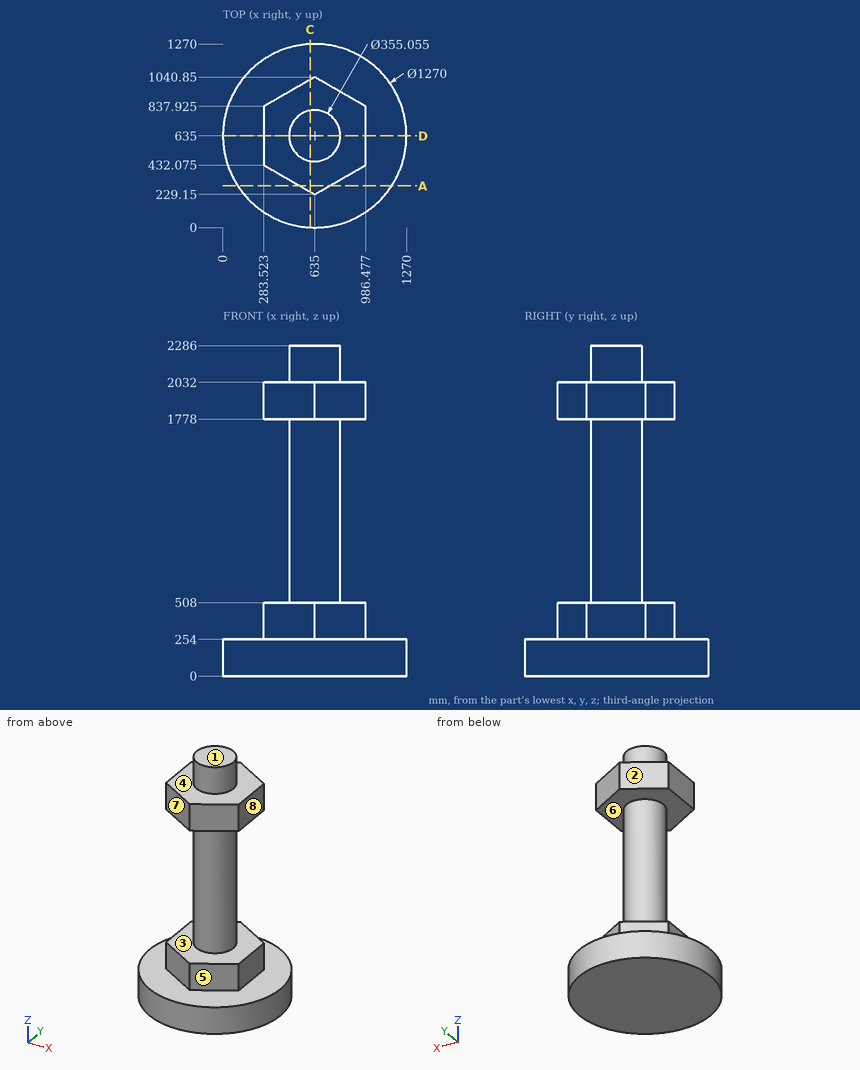
Could you check a few things on this drawing? It's one solid part, dimensions in mm from its lowest x, y, z. A direction names the side the tool comes from. Round coordinates to 2 decimals unless told otherwise and drop trailing zeros. Write each loop counter-clockwise with the first axis right and the second up, starting at its lowest first coordinate (ties: lowest second). Pieces come first, ordered by that corner, then holes. Notation, with made-up numbers: M 18.25,42 L 22.25,42 A11 cw 22.25,50 Z; hole C 41,-11.5 d5. An arc over 180 degrees is marked long. Answer as CSV lines item,"result". Start each with the question number.
1. On a 3-axis mill with a long thin cutter (end or side, diameter ignored), from which of +Z, -Z, +X, -X, +Y, -Y can I reach the whole of each face in a straight line? I mean the marked faces 4, 5, 6, 7 and 8. Say none if no direction works.
2. I need wall thicknesses on probe 1 along Z at (x, y) = (816.5, 820.5); probe 2 along X at (y, z) = (639, 1463.5); probe 3 along X at (y, z) = (620, 1981). Which ranges of each line are inside material? Lowest first, please.
3. I'm going to push a flat-ended pin straight in: pin 1 Ø8 at (x, y) = (299.5, 1017.5) entering from +Z. Where does the tip first touch, or does it pass through?
4. Suppose I cut it at C-C on x = 602.5. Write out the boundary of the cut face in (y, z).
5. Suppose I cut it at A-A on y = 288. Write out the boundary of the cut face in (x, z) (1 decimal).
6. Thinking about a two-plate mould opening in Z: for the marked faces 1, 2 and 3, which applies, released by +Z, released by -Z, zero draft, split by the parting line, or undercut?
7. Suppose I cut it at D-D on y = 635. Write out the boundary of the cut face in (x, z).
Check result:
1,face 4,"+Z"
1,face 5,"+Z, +X, -Y"
1,face 6,"none"
1,face 7,"+Z, -X, -Y"
1,face 8,"+Z, +X, +Y, -Y"
2,probe 1,"z = 0 to 508, 1778 to 2032"
2,probe 2,"x = 457.52 to 812.48"
2,probe 3,"x = 283.52 to 986.48"
3,pin 1,"stops at z = 254"
4,outline,"M 0.83,0 L 1269.17,0 L 1269.17,254 L 1022.09,254 L 1022.09,508 L 809.53,508 L 809.53,1778 L 1022.09,1778 L 1022.09,2032 L 809.53,2032 L 809.53,2286 L 460.47,2286 L 460.47,2032 L 247.91,2032 L 247.91,1778 L 460.47,1778 L 460.47,508 L 247.91,508 L 247.91,254 L 0.83,254 Z"
5,outline,"M 103.2,0 L 1166.8,0 L 1166.8,254 L 736.9,254 L 736.9,508 L 533.1,508 L 533.1,254 L 103.2,254 Z; M 533.1,1778 L 736.9,1778 L 736.9,2032 L 533.1,2032 Z"
6,face 1,"released by +Z"
6,face 2,"zero draft"
6,face 3,"undercut"
7,outline,"M 0,0 L 1270,0 L 1270,254 L 986.48,254 L 986.48,508 L 812.53,508 L 812.53,1778 L 986.48,1778 L 986.48,2032 L 812.53,2032 L 812.53,2286 L 457.47,2286 L 457.47,2032 L 283.52,2032 L 283.52,1778 L 457.47,1778 L 457.47,508 L 283.52,508 L 283.52,254 L 0,254 Z"
